Autodesk Inventor part; units mm, degrees
ref_plane "YZ Plane" through (0, 0, 0) normal (1, 0, 0) x (0, 1, 0)
ref_plane "XZ Plane" through (0, 0, 0) normal (0, 1, 0) x (-1, 0, 0)
ref_plane "XY Plane" through (0, 0, 0) normal (0, 0, 1) x (1, 0, 0)
sketch "Sketch1" plane through (0, 0, 0) normal (0, 0, 1) x (1, 0, 0)
  line L0 (-29.7451, 24.9779) -> (38.6825, 24.9779)
  line L1 (38.6825, 24.9779) -> (38.6825, -9.0073)
  line L2 (38.6825, -9.0073) -> (-29.7451, -9.0073)
  line L3 (-29.7451, -9.0073) -> (-29.7451, 24.9779)
  point P0 (0, 0)
  dimension "d0" = 68.4276
  dimension "d1" = 33.9852
extrude "Extrusion1" add sketch "Sketch1" along normal blind 18.034
fillet "Fillet1" radius 3.175 1 edges at (38.6825, 24.9779, 9.017)
fillet "Fillet2" radius 3.175 1 edges at (38.6825, -9.0073, 9.017)
properties part number "Aidan Sherry Battery Pack"
Geometry check sheet. Reference: the model listing, model coordinates, mm. Give positions to 0.01 mm unless a question says otherwise; leave off trailing zeros. One line per question, with ' | ' between items.
1. Gauge pin test, flat end, axial feed: pin 1 (10 mm diameter, centred on x = 26, y = 1.5, fed in from -Z). Record the tip position at first contact, or that the pin passes through.
Ans:
pin 1: z = 0
2. Scan line: line 1 along Y through (x, z) = (36, 13.25). Record every from-to range of solid material in increasing order. Write a range as from..to.
Ans:
line 1: -8.97..24.94
3. Mould release check, pull along X, two halves, no side actions. Record for faces 1 (the face through (3, -9.007, 9)), 2 (the face through (-29.745, 8, 9)), 3 (the face through (37.8, 24, 9.1)): released by +X, released by -X, zero draft, split by the parting line, or undercut.
Ans:
face 1: zero draft | face 2: released by -X | face 3: released by +X
